from build123d import *

# Parameters (mm, degrees)
SKETCH_1_R      = 1.5499999999999998
SKETCH_1_R_2    = 1.5499999999999994
EXTRUDE_1_DEPTH = 12
EXTRUDE_2_DEPTH = 12
FILLET_1_R      = 0.5
FILLET_2_R      = 4
FILLET_3_R      = 2


with BuildPart() as part:
    # 草图1 → 凸台-拉伸1 (new body)
    with BuildSketch(Plane.XY):
        Polygon((14.000000000000002, -2.9999999999999982), (-4.000000000000002, -3.0000000000000004), (-4.000000000000002, 4), (14.000000000000002, 4.000000000000002), align=None)
        Circle(SKETCH_1_R, mode=Mode.SUBTRACT)
        with Locations((10, 0)):
            Circle(SKETCH_1_R_2, mode=Mode.SUBTRACT)
    extrude(amount=EXTRUDE_1_DEPTH)

    # 草图2 → 凸台-拉伸2 (add)
    with BuildSketch(Plane.XY.offset(12)):
        with BuildLine():
            Line((-4.000000000000002, 4), (-4.000000000000002, -3.0000000000000004))
            Line((-4.000000000000002, -3.0000000000000004), (14.000000000000002, -2.9999999999999982))
            Line((14.000000000000002, -2.9999999999999982), (13.747325070832083, -13.216342563780504))
            ThreePointArc((13.747325070832083, -13.216342563780504), (5.32150522875723, -4.255908601356449), (-3.7395934787153213, -12.573378590451934))
            ThreePointArc((-3.7395934787153213, -12.573378590451934), (-5.421370715664583, -14.406478038174821), (-7.50358636440358, -15.767729760711498))
            Line((-7.50358636440358, -15.767729760711498), (-4.000000000000002, 4))
        make_face()
    extrude(amount=-EXTRUDE_2_DEPTH)

    # 圆角1
    fillet_1_edges = [part.edges().sort_by_distance(p)[0] for p in [
        (-7.50358636440358, -15.7677297607115, 6),
        (-3.7395934787153218, -12.573378590451934, 6),
    ]]
    fillet(fillet_1_edges, radius=FILLET_1_R)

    # 圆角2
    fillet_2_edges = [part.edges().sort_by_distance(p)[0] for p in [
        (-4.000000000000002, 4, 6),
        (14.000000000000002, 4.000000000000002, 6),
    ]]
    fillet(fillet_2_edges, radius=FILLET_2_R)

    # 圆角3
    fillet_3_edges = [part.edges().sort_by_distance(p)[0] for p in [
        (13.747325070832083, -13.216342563780504, 6),
    ]]
    fillet(fillet_3_edges, radius=FILLET_3_R)


solid = part.part
Geometry: final body of the model. Coordinates: model frame, mm. Round coordinates to 2 decimals unless told otherwise and drop trailing zeros. Order: outer loops, then holes, each group sorted by start corner. A loop starts at its lowest first (then second) coordinate and runs counter-clockwise, first axis right, second up. Notation, with made-up numbers: (-13.5, 54.5) -> (21.5, 54.5) arc R20 cw to (21.5, 72.5) -> close; hole circle Ø10 at (64.5, -6). An arc over 180 degrees is marked (long way). Put each result on its own line as item: value. Start each with the question number.
Q1. Pull-direction query (Y, two-part tool) for faces 1 (the cylindrical face through (11.432, -0.594, 5.916)), 2 (the flat face through (5, 4, 6)), 3 (the cylindrical face through (12.801, -6.615, 5.916)), 4 (the flat face through (3, -3, 12)); classes: +Y half, -Y half, draft (parallel to the pull), parting line (faces both ways), or undercut.
Q2. Line query: probe 1 along X at (y, z) = (0.5, 3); probe 2 along Y at (x, z) = (1.25, 4.75); probe 3 along Y at (x, z) = (0, 7). Output: solid intervals per line, ascending.
Q3. First-contact query: pin 1 (1.5 mm diameter, centred on x = -3.5, z = 1.5, fed in from -Y); pin 2 (10 mm diameter, centred on x = 1, y = -13.5, fed in from -Z); pin 3 (1.5 mm diameter, centred on y = -12, z = 7, fed in from -X); pin 4 (6 mm diameter, centred on x = 9.5, z = 2.5, fed in from -Y). Flat tips, straight axial feed; report the tip coordinate or a pass-through.
Q4. Section A-A on x = 0. Return the cut outline in (y, z), and give its area (3 significant figures).
Q5. Section C-C on z = 8.75. Give the number of separate pieces and of enclosed holes in the cut face, and give its area (4 significant figures).
Q6. Section B-B on y = -5.5. Return the cut outline in (x, z).
Q7. Section D-D on x = 12.5. Return the cut outline in (y, z).
Ans:
1. face 1: undercut
1. face 2: +Y half
1. face 3: -Y half
1. face 4: draft
2. probe 1: x = -4.62 to -1.47, 1.47 to 8.53, 11.47 to 13.97
2. probe 2: y = -5.09 to -0.92, 0.92 to 4
2. probe 3: y = -5.82 to -1.55, 1.55 to 4
3. pin 1: stops at y = -13.23
3. pin 2: stops at z = 0
3. pin 3: stops at x = -6.97
3. pin 4: stops at y = -6.8
4. outline: (-5.82, 0) -> (-1.55, 0) -> (-1.55, 12) -> (-5.82, 12) -> close; (1.55, 0) -> (4, 0) -> (4, 12) -> (1.55, 12) -> close
4. area: 80.6 mm2
5. separate pieces: 1
5. enclosed holes: 2
5. area: 187.5 mm2
6. outline: (-5.68, 0) -> (0.49, 0) -> (0.49, 12) -> (-5.68, 12) -> close; (9.51, 0) -> (13.83, 0) -> (13.83, 12) -> (9.51, 12) -> close
7. outline: (-6.73, 0) -> (3.12, 0) -> (3.12, 12) -> (-6.73, 12) -> close
